from build123d import *

# Parameters (mm, degrees)
F1_DEPTH = 15.494


with BuildPart() as f1:
    # F0 (on Front) → F1 (new body)
    with BuildSketch(Plane.XZ):
        Polygon((-34.167524, 30.66401), (-51.991723, -38.114682), (-5.041494, -37.326522), (-11.365365, 12.815122), (-13.61647, 30.66401), align=None)
        Polygon((12.548127, 30.66401), (-13.61647, 30.66401), (-11.365365, 12.815122), (12.548127, 12.815122), align=None)
    extrude(amount=-F1_DEPTH)


solid = f1.part
Check sheet for the modelled part. Datum: model origin and axes. Units: mm. A direction names the side the tool comes from. Round coordinates to 2 decimals unless told otherwise and drop trailing zeros. Write each loop counter-clockwise with the first axis right and the second up, starting at its lowest first coordinate (ties: lowest second). Pieces come first, ordered by that corner, then holes. Notation, with made-up numbers: (-23, 64.5) - (-18, 64.5) arc R19 cw to (-18, 68.5) - close; hole circle Ø6 at (19, 22). An arc over 180 degrees is marked (long way). Return JSON: item names as keys, results as strings.
Q1. Depth check by flat-ended pin: P1, Ø1, axis at y = 10, z = 20, coming from the -X side; P2, Ø3, axis at y = 11.5, z = 6, coming from the +X side; P3, Ø4, axis at y = 2, z = -5, coming from the -X side. Enter the tip coordinate at first touch or a pass-through.
Returned:
{"P1": "stops at x = -37.06", "P2": "stops at x = -10.32", "P3": "stops at x = -43.93"}
Q2. Cross-section at A-A (x = -10.5). Record the boundary of the cut face in (y, z), then the cut area to 3 significant figures.
Returned:
{"outline": "(0, -37.42) - (15.49, -37.42) - (15.49, 5.95) - (0, 5.95) - close; (0, 12.82) - (15.49, 12.82) - (15.49, 30.66) - (0, 30.66) - close", "area": "949 mm²"}
Q3. Scan lines: L1, parallel to Z at x = 9.5, y = 12.25; L2, parallel to X at y = 10.5, z = 15.5; L3, parallel to X at y = 5.75, z = 14. Record each from-to range of solid material in increasing order. Write a range as from..to.
Returned:
{"L1": "z = 12.82..30.66", "L2": "x = -38.1..12.55", "L3": "x = -38.49..12.55"}
Q4. Cross-section at B-B (y = 10). Record the boundary of the cut face in (x, z).
Returned:
{"outline": "(-51.99, -38.11) - (-5.04, -37.33) - (-11.37, 12.82) - (12.55, 12.82) - (12.55, 30.66) - (-34.17, 30.66) - close"}
Q5. Draft check along Z on faces 1 (the flat face through (-42.955, 7.639, -3.244)), 2 (the flat face through (-20, 0, -3)), 3 (the flat face through (-8.16, 7.64, -12.61)). Enter one of: released by +Z, released by -Z, zero draft, split by the parting line, or undercut.
Returned:
{"face 1": "released by +Z", "face 2": "zero draft", "face 3": "undercut"}
Q6. Access from +Z, -Z, +X, -X, +Y, -Y to the whole of each face (thin tool, end or side, straight path). Record for faces 4 (the flat face through (-10, 8, 30.664)), 5 (the flat face through (0, 8, 12.815)).
Returned:
{"face 4": "+Z, +X, -X, +Y, -Y", "face 5": "+X, +Y, -Y"}
Q7. Cross-section at D-D (x = -2). Record the boundary of the cut face in (y, z).
Returned:
{"outline": "(0, 12.82) - (15.49, 12.82) - (15.49, 30.66) - (0, 30.66) - close"}
Q8. Cross-section at C-C (z = 6.5). Record the boundary of the cut face in (x, y), then the cut area to 3 significant figures.
Returned:
{"outline": "(-40.43, 0) - (-10.57, 0) - (-10.57, 15.49) - (-40.43, 15.49) - close", "area": "463 mm²"}
